Read the model definition and answer for the solid it produces. Units are mm, in the model's axes. A direction names the side the tool comes from. Give positions to 0.01 mm unless a question says otherwise; leave off trailing zeros. Loops run counter-clockwise (first coordinate to the right, second up) from the corner with the lowest first, then second, coordinate; pieces in that order, holes last. Notation, with made-up numbers: (20, -34) -> (71, -34) arc R21 cw to (71, -30) -> close; hole circle Ø1 at (6, 1). An arc over 180 degrees is marked (long way). Write each question's results on one line, items separated by ' | '. Start each with the question number.
Item 1: Find the intervals of material crossed by line 1 (X direction, y = 5, z = 5.75); line 2 (X direction, y = 3.25, z = 3.5); line 3 (Z direction, x = 2, y = 2.25), in increasing order.
Item 2: Section C-C on y = 13.75 is taken. Write down the section's boundary in (x, z), and give its area (3 significant figures).
Item 3: Section D-D on x = 3 is taken. Write down the section's boundary in (y, z), and give its area (3 significant figures).
Item 4: Section B-B on z = -0.5 is taken. Write down the section's boundary in (x, y).
Item 5: Determine the mould class of faces 5 (the flat face through (-4.99, 11, 6)), 6 (the flat face through (-6, 11, 12.5)), 7 (the flat face through (-6.99, 15, 5)) for opening direction X: +X half, -X half, draft (parallel to the pull), parting line (faces both ways), or undercut.
Item 6: Each of these flat-tipped pins is pushed along its axis until it touches: P1, Ø1.5, axis at x = -8.5, z = 4, coming from the -Y side; P2, Ø1, axis at x = -3, y = 6, coming from the +Z side; P3, Ø7, axis at y = 13.5, z = 8, coming from the +X side. Where does it stop, or does it pass through?
Item 7: Which of the six approach directions +Z, -Z, +X, -X, +Y, -Y give full straight-line access (tool end or side, diameter ignored) to faces 1 (the flat face through (-8, 4, 5)), 2 (the flat face through (4.99, 11, 6)), 3 (the flat face through (8, 4, 5)), 4 (the flat face through (8, 7, 5))?
Item 8: Section A-A on z = 9.5 is taken. Write down the section's boundary in (x, y), and give its area (3 significant figures).
```python
from build123d import *

# Parameters (mm, degrees)
BOSS_EXTRUDE1_DEPTH = 23
SKETCH9_W           = 14.5
SKETCH9_H           = 3
BOSS_EXTRUDE4_DEPTH = 3


with BuildPart() as part:
    # Sketch1 → Boss-Extrude1 (new body)
    with BuildSketch(Plane(origin=(0, 0, 0), x_dir=(1, 0, 0), z_dir=(0, 1, 0))):
        Polygon((-4.99, 0), (4.99, 0), (4.99, -12.5), (6.99, -12.5), (6.99, 2), (-6.99, 2), (-6.99, -12.5), (-4.99, -12.5), align=None)
    extrude(amount=BOSS_EXTRUDE1_DEPTH)

    # Sketch9 → Boss-Extrude4 (add)
    with BuildSketch(Plane.ZY.offset(6.99)):
        with Locations((5.25, 5.5)):
            Rectangle(SKETCH9_W, SKETCH9_H)
    boss_extrude4 = extrude(amount=BOSS_EXTRUDE4_DEPTH)

    # Mirror1: Boss-Extrude4 across plane
    add(boss_extrude4.mirror(Plane.ZY))


solid = part.part
```
Findings:
1) line 1: -9.99 to -4.99, 4.99 to 9.99 | line 2: -6.99 to -4.99, 4.99 to 6.99 | line 3: -2 to 0
2) outline: (-6.99, -2) -> (6.99, -2) -> (6.99, 12.5) -> (4.99, 12.5) -> (4.99, 0) -> (-4.99, 0) -> (-4.99, 12.5) -> (-6.99, 12.5) -> close | area: 78.0 mm2
3) outline: (0, -2) -> (23, -2) -> (23, 0) -> (0, 0) -> close | area: 46.0 mm2
4) outline: (-9.99, 4) -> (-6.99, 4) -> (-6.99, 0) -> (6.99, 0) -> (6.99, 4) -> (9.99, 4) -> (9.99, 7) -> (6.99, 7) -> (6.99, 23) -> (-6.99, 23) -> (-6.99, 7) -> (-9.99, 7) -> close
5) face 5: undercut | face 6: draft | face 7: -X half
6) P1: y = 4 | P2: z = 0 | P3: x = 6.99
7) face 1: +Z, -Z, -X, -Y | face 2: +Z, +Y, -Y | face 3: +Z, -Z, +X, -Y | face 4: +Z, -Z, +X, +Y
8) outline: (-9.99, 4) -> (-6.99, 4) -> (-6.99, 0) -> (-4.99, 0) -> (-4.99, 23) -> (-6.99, 23) -> (-6.99, 7) -> (-9.99, 7) -> close; (4.99, 0) -> (6.99, 0) -> (6.99, 4) -> (9.99, 4) -> (9.99, 7) -> (6.99, 7) -> (6.99, 23) -> (4.99, 23) -> close | area: 110 mm2
